Autodesk Inventor part; units mm, degrees
ref_plane "Work Plane2" through (0, 1.5, -4) normal (0, 0, 1) x (1, 0, 0)
ref_plane "YZ Plane" through (0, 0, 0) normal (1, 0, 0) x (0, 1, 0)
ref_plane "XZ Plane" through (0, 0, 0) normal (0, 1, 0) x (-1, 0, 0)
sketch "Sketch11" plane through (0, 0, 0) normal (0, 0, 1) x (1, 0, 0)
  line L0 (0, 0) -> (0, 6)
  line L1 (-4, 0) -> (-4, 3)
  line L2 (-4, 3) -> (-22.5, 3)
  line L3 (-22.5, 3) -> (-22.5, 6)
  line L4 (-22.5, 6) -> (-1.5, 6)
  line L5 (-1.5, 6) -> (-1.5, 0)
  line L6 (-1.5, 0) -> (-4, 0)
  dimension "d59" = 3
  dimension "d60" = 6
  dimension "d61" = 3
  dimension "d62" = 45
  dimension "d63" = 2.5
revolve "Revolution3" add sketch "Sketch11" angle 360 about axis through (0, 0, 0) along (0, 1, 0)
sketch "Sketch12" plane through (0, 6, 0) normal (0, 1, 0) x (1, 0, 0)
  circle A0 centre (1.7213, -19.6748) radius 1
  circle A1 centre (-1.7213, -19.6748) radius 1
  circle A2 centre (-5.1117, -19.077) radius 1
  circle A3 centre (5.1117, -19.077) radius 1
  circle A4 centre (0, 0) radius 19.75 construction
  line L0 (0, 0) -> (0, -19.75) construction
  line L1 (0, 0) -> (-1.7213, -19.6748) construction
  line L2 (0, 0) -> (-5.1117, -19.077) construction
  line L3 (0, 0) -> (1.7213, -19.6748) construction
  line L4 (0, 0) -> (5.1117, -19.077) construction
  line L5 (-5.1117, -19.077) -> (-1.7213, -19.6748) construction
  line L6 (-1.7213, -19.6748) -> (1.7213, -19.6748) construction
  dimension "d65" = 2
  dimension "d66" = 2
  dimension "d67" = 2
  dimension "d68" = 2
  dimension "d71" = 5
  dimension "d72" = 10
  dimension "d73" = 10
  dimension "d81" = 39.5
  dimension "d90" = 10.2233
extrude "Extrusion7" cut sketch "Sketch12" against normal through all
sketch "Sketch14" plane through (0, 6, 0) normal (0, 1, 0) x (1, 0, 0)
  circle A0 centre (0, 0) radius 22.5
  line L0 (0, 0) -> (0, -22.5)
  line L1 (0, 0) -> (-8.4286, -20.8616)
  line L2 (0, 0) -> (8.4286, -20.8616)
  circle A1 centre (0, 0) radius 4
  point P0 (1.4984, -3.7087)
  point P1 (-1.4984, -3.7087)
  dimension "d76" = 22
  dimension "d77" = 22
extrude "Extrusion8" cut sketch "Sketch14" against normal through all contours A0 L2 A1 L1
fillet "Fillet3" radius 3 2 edges at (8.4286, 4.5, 20.8616) (-8.4286, 4.5, 20.8616)
fillet "Fillet4" radius 8 2 edges at (1.4984, 4.5, 3.7087) (-1.4984, 4.5, 3.7087)
ref_plane "Work Plane2" through (0, 1.5, -4) normal (0, 0, 1) x (1, 0, 0)
sketch "Sketch15" plane through (0, 1.5, -4) normal (0, 0, 1) x (1, 0, 0)
  line L0 (4, 4.5) -> (-4, 4.5)
  line L1 (4, -1.5) -> (4, 4.5)
  point P0 (0, -1.5)
  point P1 (0, 1.5)
  point P2 (3.5894, 4.5)
  point P3 (-3.5894, 4.5)
  point P4 (0, 4.5)
  point P5 (4, 1.5)
hole "Hole3" at (0, 3, -4) direction (0, 0, 1) diameter 1.567 depth 4.5 tip angle 118
equation "\"d71\" = 0.5 * d72"
equation "\"d73\" = d72"
equation "\"d77\" = d76"
properties part number "023" material "Stainless Steel, Austenitic"
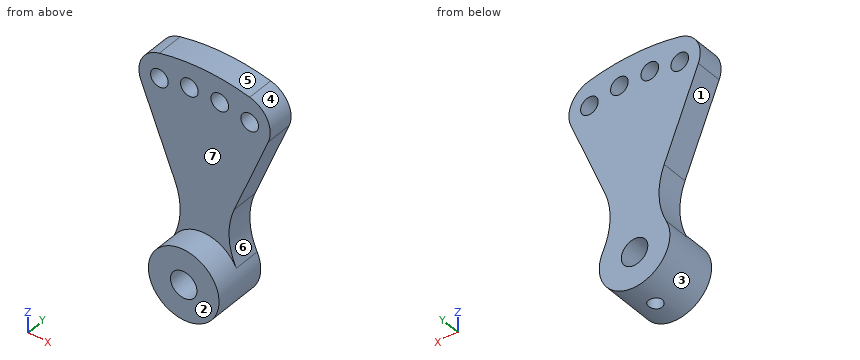
For this review, take the finished solid that the model builds, in its own axes (mm). Face numbers are marked on the shaded views. A direction names the side the tool comes from. Round coordinates to 2 decimals unless told otherwise and drop trailing zeros. Loops run counter-clockwise (first coordinate to the right, second up) from the corner with the lowest first, then second, coordinate; pieces in that order, holes last.
Q1. Insertion check: pin 1 Ø1.5 at (x, z) = (2.5, 6) entering from -Y. The pin has a flat end and moves straight along its axis. Give the tip position at first contact, or say it passes through.
Result sheet:
pin 1: stops at y = 3
Q2. Machinability: for the marked faces 1, 2 and 3, which of the approach directions +Z, -Z, +X, -X, +Y, -Y give a long, thin tool a straight path to every point of the face, cutting with its end or side? Answer none if there is none.
Result sheet:
face 1: -X, +Y, -Y
face 2: +Z, -Z, +X, -X, -Y
face 3: -Y
Q3. Add section C-C on y = 1.25. Write out the cut boundary in (x, z).
Result sheet:
outline: circle Ø8 at (0, 0); hole circle Ø3 at (0, 0)
Q4. To check wall thickness, follow line 1 along Y through (x, z) = (2, 7.5); line 2 along Z through (x, y) = (-5.5, 4.75); line 3 along Z through (x, y) = (-1.75, 0.75). State the ranges of each line that lie inside material, in increasing order.
Result sheet:
line 1: y = 3 to 6
line 2: z = 13.61 to 18.16, 20 to 21.79
line 3: z = -3.6 to 3.6
Q5. Mouldability with a two-part tool opening along Z and no side actions: class the marked faces 4, 5, 6 and 7 as +Z half, -Z half, draft (parallel to the pull), parting line (faces both ways), or undercut.
Result sheet:
face 4: parting line
face 5: +Z half
face 6: undercut
face 7: draft
Q6. Add section D-D on y = 4.5. Write out the cut boundary in (x, z).
Result sheet:
outline: (-7.22, 17.86) - (-3.35, 8.29) arc R8 cw to (-3.59, 1.77) arc R4 ccw (long way) to (3.59, 1.77) arc R8 cw to (3.35, 8.29) - (7.22, 17.86) arc R3 ccw to (5.12, 21.91) arc R22.5 ccw to (-5.12, 21.91) arc R3 ccw to start; hole circle Ø2 at (-5.11, 19.08); hole circle Ø2 at (-1.72, 19.67); hole circle Ø3 at (0, 0); hole circle Ø2 at (1.72, 19.67); hole circle Ø2 at (5.11, 19.08)
Q7. Add section A-A on x = 0. Write out the cut boundary in (y, z).
Result sheet:
outline: (0, -4) - (2.22, -4) - (2.22, -1.5) - (0, -1.5) - close; (0, 1.5) - (6, 1.5) - (6, 22.5) - (3, 22.5) - (3, 4) - (0, 4) - close; (3.78, -4) - (6, -4) - (6, -1.5) - (3.78, -1.5) - close
Q8. Add section B-B on x = 2. Write out the cut boundary in (y, z), plus the area to 3 significant figures.
Result sheet:
outline: (0, -3.46) - (6, -3.46) - (6, 18.71) - (3, 18.71) - (3, 3.46) - (0, 3.46) - close; (3, 20.64) - (6, 20.64) - (6, 22.41) - (3, 22.41) - close
area: 92.6 mm2
